Design review of the part built by this model. Coordinates are the model's own, in mm. Round coordinates to 2 decimals unless told otherwise and drop trailing zeros. Order: outer loops, then holes, each group sorted by start corner. A loop starts at its lowest first (then second) coordinate and runs counter-clockwise, first axis right, second up. Notation, with made-up numbers: (22, 49) - (38, 49) arc R29 ccw to (38, 82) - close; hole circle Ø8 at (10, 27). An arc over 180 degrees is marked (long way). Write item = value, one per line.
Autodesk Inventor part; units mm, degrees
ref_plane "YZ Plane" through (0, 0, 0) normal (1, 0, 0) x (0, 1, 0)
ref_plane "XZ Plane" through (0, 0, 0) normal (0, 1, 0) x (-1, 0, 0)
ref_plane "XY Plane" through (0, 0, 0) normal (0, 0, 1) x (1, 0, 0)
sketch "Sketch1" plane through (0, 0, 0) normal (0, 1, 0) x (-1, 0, 0)
  line L0 (-111.8414, 23.1497) -> (72.3086, 23.1497)
  line L1 (72.3086, 23.1497) -> (72.3086, -148.2749)
  line L2 (72.3086, -148.2749) -> (-111.8414, 23.1497)
  circle A0 centre (62.7836, 13.6247) radius 3.3528
  circle A1 centre (-89.6164, 13.6247) radius 3.3566
  line L3 (-99.1414, 23.1497) -> (-99.1414, 11.3273)
  line L4 (38.6383, -116.9313) -> (72.3086, -116.9313)
  point P0 (0, 0)
  dimension "d0" = 184.15
  dimension "d1" = 171.4246
  dimension "d2" = 6.7056
  dimension "d3" = 9.525
  dimension "d4" = 6.7132
  dimension "d5" = 152.4
  dimension "d8" = 12.7
  dimension "d9" = 9.525
  dimension "d10" = 140.081
extrude "Extrusion1" add sketch "Sketch1" along normal blind 12.7 contours L0 L1 L4 L2 L3
properties part number "BallGuidePlyRight"
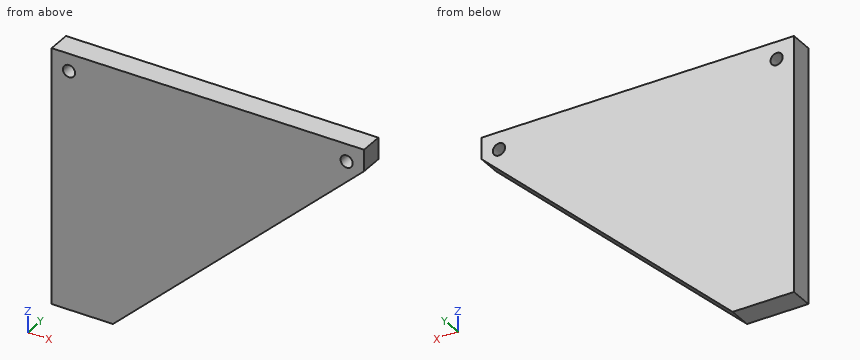
Item 1: Take a section at A-A, the plane y = 10. State the section outline as (x, z) points.
Data:
outline = (-72.31, -116.93) - (-38.64, -116.93) - (99.14, 11.33) - (99.14, 23.15) - (-72.31, 23.15) - close; hole circle Ø6.71 at (-62.78, 13.62); hole circle Ø6.71 at (89.62, 13.62)
Item 2: Take a section at C-C, the plane x = 25.5. State the section outline as (y, z) points.
Data:
outline = (0, -57.23) - (12.7, -57.23) - (12.7, 23.15) - (0, 23.15) - close
Item 3: Take a section at B-B, the plane z = -9. State the section outline as (x, y) points, and give its area (3 significant figures).
Data:
outline = (-72.31, 0) - (77.31, 0) - (77.31, 12.7) - (-72.31, 12.7) - close
area = 1,900 mm2
Item 4: For line 1 along X through (y, z) = (12, 14); line 2 along Z through (x, y) = (-63, 7.75); line 3 along X through (y, z) = (1.5, -41.5), list the stretches that pass through material, from the lowest coordinate up. Write a range as [from, to].
Data:
line_1 = [-72.31, -66.12], [-59.45, 86.28], [92.95, 99.14]
line_2 = [-116.93, 10.28], [16.97, 23.15]
line_3 = [-72.31, 42.39]
Item 5: Insertion check: P1, Ø3, axis at y = 8, z = -59, coming from the +X side; P2, Ø5.5, axis at x = -62.78, z = 13.62, coming from the +Y side; P3, Ø8.5, axis at x = 89.62, z = 13.62, coming from the -Y side. Each pin has a flat end and moves straight along its axis. Give the tip position at first contact, or say it passes through.
Data:
P1 = 25.2
P2 = through
P3 = 0
